```python
from build123d import *

# Parameters (mm, degrees)
F0_R     = 3.5
F1_DEPTH = 2.5


with BuildPart() as f1:
    # F0 (on Top) → F1 (new body)
    with BuildSketch(Plane.XY):
        with BuildLine():
            Line((-60.635068, 58.814), (-63.489865, 58.814))
            ThreePointArc((-63.489865, 58.814), (-67.297148, 57.055079), (-68.425747, 53.015837))
            Line((-68.425747, 53.015837), (-51.185882, -53.596367))
            ThreePointArc((-51.185882, -53.596367), (-49.491079, -56.605488), (-46.25, -57.798204))
            Line((-46.25, -57.798204), (46.25, -57.798204))
            ThreePointArc((46.25, -57.798204), (50.057284, -56.039283), (51.185882, -52.000041))
            Line((51.185882, -52.000041), (46.832282, -25.077153))
            ThreePointArc((46.832282, -25.077153), (45.910862, -22.894697), (44.088255, -21.381346))
            Line((44.088255, -21.381346), (35.013699, -16.955389))
            ThreePointArc((35.013699, -16.955389), (31.501043, -16.626965), (28.645966, -18.699441))
            ThreePointArc((28.645966, -18.699441), (-19.4939, -27.679928), (-26.675491, 20.760971))
            ThreePointArc((-26.675491, 20.760971), (-25.645449, 24.135231), (-27.099589, 27.349589))
            Line((-27.099589, 27.349589), (-57.099534, 57.349534))
            ThreePointArc((-57.099534, 57.349534), (-58.721651, 58.433398), (-60.635068, 58.814))
        make_face()
        with Locations((-46.25, -52.798204)):
            Circle(F0_R, mode=Mode.SUBTRACT)
        with Locations((-13.75, -42)):
            Circle(F0_R, mode=Mode.SUBTRACT)
        with Locations((14.25, -42)):
            Circle(F0_R, mode=Mode.SUBTRACT)
        with Locations((46.25, -52.798204)):
            Circle(F0_R, mode=Mode.SUBTRACT)
        with Locations((-63.489865, 53.814)):
            Circle(F0_R, mode=Mode.SUBTRACT)
    extrude(amount=F1_DEPTH)


solid = f1.part
```
The listing builds one solid part. Answer for the finished solid, in the listing's coordinates (mm). Round coordinates to 2 decimals unless told otherwise and drop trailing zeros. Loops run counter-clockwise (first coordinate to the right, second up) from the corner with the lowest first, then second, coordinate; pieces in that order, holes last.
Q1. Find the intervals of material crossed by line 1 (X direction, y = 53, z = 0.75); line 2 (Y direction, x = 33, z = 0.55); line 3 (Y direction, x = 46, z = 1.75), in increasing order.
Q2. Section A-A, the plane x = -12.5 is taken. Determine the outline of the cut face in (y, z).
Q3. Section D-D, the plane x = 0.25 is taken. Determine the outline of the cut face in (y, z).
Q4. Given pin 1 Ø8 at (x, y) = (-63.49, 53.81) entering from -Z; pin 2 Ø3 at (x, y) = (-22.5, 26) entering from -Z; pin 3 Ø1.5 at (x, z) = (0, 2) entering from +Y, each flat-ended and moving along its own axis, determine where each tip first touches the part or whether it passes through.
Q5. Section B-B, the plane y = -42 is taken. Determine the outline of the cut face in (x, z).
Q6. Section C-C, the plane z = 1.2 is taken. Determine the outline of the cut face in (x, y).
Q7. For a pull along Y with two mould halves and no side action, classify faces 1 (the face through (-41.89, 42.14, 1.23)), 2 (the face through (13.79, -38.53, 1.23)), 3 (the face through (-36, -25, 0)), 4 (the face through (-14.21, -38.53, 1.23)) as released by +Y, released by -Y, zero draft, split by the parting line, or undercut.
Completed:
1. line 1: x = -68.42 to -66.89, -60.09 to -52.75
1. line 2: y = -57.8 to -16.45
1. line 3: y = -57.8 to -56.29, -49.31 to -23.02
2. outline: (-57.8, 0) - (-45.27, 0) - (-45.27, 2.5) - (-57.8, 2.5) - close; (-38.73, 0) - (-31.52, 0) - (-31.52, 2.5) - (-38.73, 2.5) - close
3. outline: (-57.8, 0) - (-34, 0) - (-34, 2.5) - (-57.8, 2.5) - close
4. pin 1: stops at z = 0
4. pin 2: passes through
4. pin 3: stops at y = -33.99
5. outline: (-53.06, 0) - (-17.25, 0) - (-17.25, 2.5) - (-53.06, 2.5) - close; (-10.25, 0) - (10.75, 0) - (10.75, 2.5) - (-10.25, 2.5) - close; (17.75, 0) - (49.57, 0) - (49.57, 2.5) - (17.75, 2.5) - close
6. outline: (-68.43, 53.02) - (-51.19, -53.6) arc R5 ccw to (-46.25, -57.8) - (46.25, -57.8) arc R5 ccw to (51.19, -52) - (46.83, -25.08) arc R5 ccw to (44.09, -21.38) - (35.01, -16.96) arc R5 ccw to (28.65, -18.7) arc R34 cw (long way) to (-26.68, 20.76) arc R5 ccw to (-27.1, 27.35) - (-57.1, 57.35) arc R5 ccw to (-60.64, 58.81) - (-63.49, 58.81) arc R5 ccw to start; hole circle Ø7 at (-63.49, 53.81); hole circle Ø7 at (-46.25, -52.8); hole circle Ø7 at (-13.75, -42); hole circle Ø7 at (14.25, -42); hole circle Ø7 at (46.25, -52.8)
7. face 1: released by +Y
7. face 2: undercut
7. face 3: zero draft
7. face 4: undercut
